Can you work these out from the drawing? Everything is in mm from the part's minimum corner. A direction names the side the tool comes from. Give positions to 0.01 mm unless a question says otherwise; leave off trailing zeros. Write each loop counter-clockwise with the first axis right and the second up, starting at its lowest first coordinate (ties: lowest second). Pieces come first, ordered by that corner, then holes. Notation, with made-up numbers: (29, 80) - (57, 80) arc R22 ccw to (57, 91) - close; hole circle Ø8 at (34.25, -5.75). An arc over 180 degrees is marked (long way). Use a Markdown table: item, result.
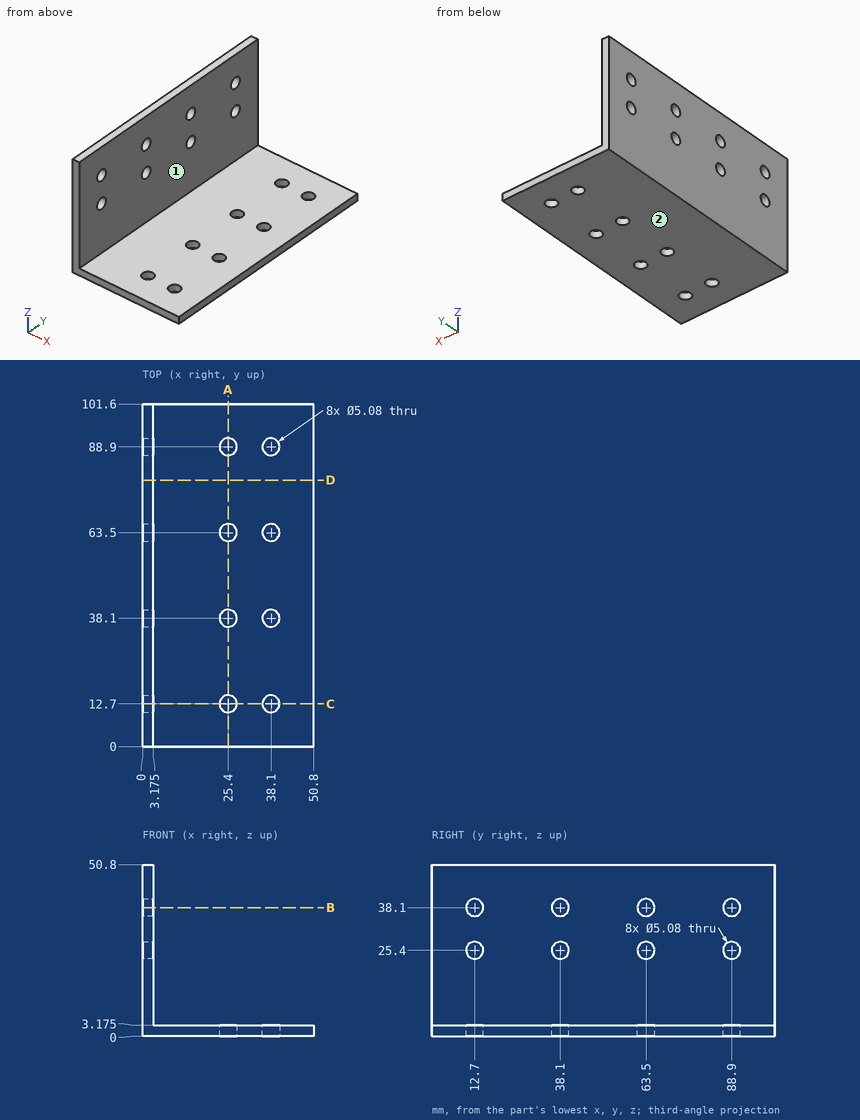
Item 1: If we section it at D-D, the plane y = 79: Write out the boundary of the cut face in (x, z) (3 decimals).
Values:
| item | result |
|---|---|
| outline | (0, 0) - (50.8, 0) - (50.8, 3.175) - (3.175, 3.175) - (3.175, 50.8) - (0, 50.8) - close |
Item 2: If we section it at B-B, the plane z = 38.1: Write out the boundary of the cut face in (x, y) (3 decimals), plus the area to 3 significant figures.
Values:
| item | result |
|---|---|
| outline | (0, 0) - (3.175, 0) - (3.175, 10.16) - (0, 10.16) - close; (0, 15.24) - (3.175, 15.24) - (3.175, 35.56) - (0, 35.56) - close; (0, 40.64) - (3.175, 40.64) - (3.175, 60.96) - (0, 60.96) - close; (0, 66.04) - (3.175, 66.04) - (3.175, 86.36) - (0, 86.36) - close; (0, 91.44) - (3.175, 91.44) - (3.175, 101.6) - (0, 101.6) - close |
| area | 258 mm2 |
Item 3: If we section it at C-C, the plane y = 12.7: Write out the boundary of the cut face in (x, z) (3 decimals), plus the area to 3 significant figures.
Values:
| item | result |
|---|---|
| outline | (0, 0) - (22.86, 0) - (22.86, 3.175) - (3.175, 3.175) - (3.175, 22.86) - (0, 22.86) - close; (0, 27.94) - (3.175, 27.94) - (3.175, 35.56) - (0, 35.56) - close; (0, 40.64) - (3.175, 40.64) - (3.175, 50.8) - (0, 50.8) - close; (27.94, 0) - (35.56, 0) - (35.56, 3.175) - (27.94, 3.175) - close; (40.64, 0) - (50.8, 0) - (50.8, 3.175) - (40.64, 3.175) - close |
| area | 248 mm2 |
Item 4: If we section it at A-A, the plane x = 25.4: Write out the boundary of the cut face in (y, z) (3 decimals), plus the area to 3 significant figures.
Values:
| item | result |
|---|---|
| outline | (0, 0) - (10.16, 0) - (10.16, 3.175) - (0, 3.175) - close; (15.24, 0) - (35.56, 0) - (35.56, 3.175) - (15.24, 3.175) - close; (40.64, 0) - (60.96, 0) - (60.96, 3.175) - (40.64, 3.175) - close; (66.04, 0) - (86.36, 0) - (86.36, 3.175) - (66.04, 3.175) - close; (91.44, 0) - (101.6, 0) - (101.6, 3.175) - (91.44, 3.175) - close |
| area | 258 mm2 |
Item 5: Will these pins go through, and if not, where does the flat tip stop? pin 1 Ø8 at (y, z) = (88.9, 25.4) entering from -X; pin 2 Ø4 at (x, y) = (27.5, 18) entering from +Z (3 decimals); pin 3 Ø5 at (y, z) = (71.5, 18) entering from +X (3 decimals).
Values:
| item | result |
|---|---|
| pin 1 | stops at x = 0 |
| pin 2 | stops at z = 3.175 |
| pin 3 | stops at x = 3.175 |
Item 6: I need wall thicknesses on line 1 along Y through (x, z) = (1, 38); line 2 along X through (y, z) = (69, 22.5) (3 decimals). Which ranges of each line are inside material? Lowest first, please. Write a range as [from, to].
Values:
| item | result |
|---|---|
| line 1 | y = [0, 10.16], [15.24, 35.56], [40.64, 60.96], [66.04, 86.36], [91.44, 101.6] |
| line 2 | x = [0, 3.175] |
Item 7: For the marked faces 1 and 2, which set-ups out of +Z, -Z, +X, -X, +Y, -Y let a thin tool reach every point of the face, with its end or its side?
Values:
| item | result |
|---|---|
| face 1 | +Z, +X, +Y, -Y |
| face 2 | -Z, +X, -X, +Y, -Y |
